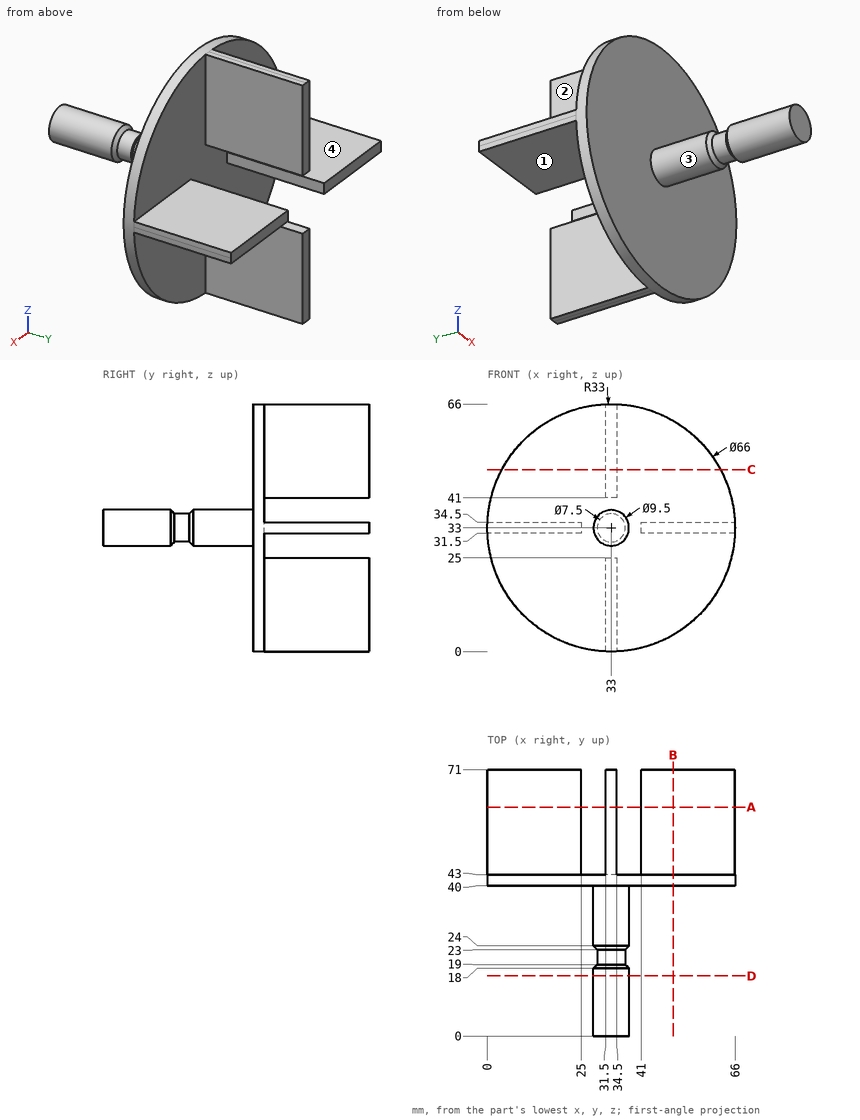
Design review of the part shown in the three views and the two pictorial views. Dimensions are in mm from the part's minimum x, y and z. A direction names the side the tool comes from. Round coordinates to 2 decimals unless told otherwise and drop trailing zeros. Write each loop counter-clockwise with the first axis right and the second up, starting at its lowest first coordinate (ties: lowest second). Pieces come first, ordered by that corner, then holes. Notation, with made-up numbers: (15, 85) -> (29, 85) arc R17 ccw to (29, 97) -> close; hole circle Ø5 at (-28, 35.25). An arc over 180 degrees is marked (long way). Write item = value, one per line. Start each with the question number.
1) Take a section at D-D, the plane y = 16. State the section outline as (x, z) points.
2) Wall thickness on probe 1 along Y at (x, z) = (21.5, 10); probe 2 along Z at (x, y) = (7, 51.5): over which ranges is each line inside the solid? List them lowest first. Write a range as from..to.
3) Clearance check with flat-ended pins moving along their axes: pin 1 (7.5 mm diameter, centred on x = 17, y = 63, fed in from -Z); pin 2 (1 mm diameter, centred on x = 14, z = 43.5, fed in from +Y); pin 3 (7.5 mm diameter, centred on y = 57.5, z = 48.5, fed in from -X). State where each tip first meets the part, or that it passes through.
4) Take a section at B-B, the plane x = 49.5. State the section outline as (y, z) points, plus the area to 3 significant figures.
5) Tool access review of the marked faces 1, 2, 3 and 4: name each direction out of +Z, -Z, +X, -X, +Y, -Y from which nothing blocks a thin tool from reaching the whole face with its end or side.
6) Take a section at A-A, the plane y = 61. State the section outline as (x, z) points.
7) Take a section at C-C, the plane z = 48.5. State the section outline as (x, y) points, plus the area to 3 significant figures.
Results list:
q1.outline = circle Ø9.5 at (33, 33)
q2.probe_1 = 40..43
q2.probe_2 = 31.5..34.5
q3.pin_1 = 31.5
q3.pin_2 = 43
q3.pin_3 = 31.5
q4.outline = (40, 4.42) -> (43, 4.42) -> (43, 31.5) -> (71, 31.5) -> (71, 34.5) -> (43, 34.5) -> (43, 61.58) -> (40, 61.58) -> close
q4.area = 255 mm²
q5.face_1 = -Z, +X, -X, +Y
q5.face_2 = +Z, -Z, -X, +Y
q5.face_3 = -Y
q5.face_4 = +Z, +X, -X, +Y
q6.outline = (0.03, 31.5) -> (25, 31.5) -> (25, 34.5) -> (0.03, 34.5) arc R33 ccw to start; (31.5, 0.03) arc R33 ccw to (34.5, 0.03) -> (34.5, 25) -> (31.5, 25) -> close; (31.5, 41) -> (34.5, 41) -> (34.5, 65.97) arc R33 ccw to (31.5, 65.97) -> close; (41, 31.5) -> (65.97, 31.5) arc R33 ccw to (65.97, 34.5) -> (41, 34.5) -> close
q7.outline = (3.87, 40) -> (62.13, 40) -> (62.13, 43) -> (34.5, 43) -> (34.5, 71) -> (31.5, 71) -> (31.5, 43) -> (3.87, 43) -> close
q7.area = 259 mm²
